Design review of the part built by this model. Coordinates are the model's own, in mm. Give positions to 0.01 mm unless a question says otherwise; leave off trailing zeros. Loops run counter-clockwise (first coordinate to the right, second up) from the corner with the lowest first, then second, coordinate; pieces in that order, holes last. Notation, with made-up numbers: M 61.5,-8.5 L 74.5,-8.5 A26 ccw 74.5,24.5 Z; hole C 27.5,35.25 d1. An arc over 180 degrees is marked long. Use one line per item in the form item = value. Start each with the question number.
from build123d import *

# Parameters (mm, degrees)
SKETCH1_W           = 25.4
SKETCH1_H           = 25.4
BOSS_EXTRUDE1_DEPTH = 3.175
CUT_EXTRUDE1_REACH  = 5.175
SKETCH2_R           = 2.5527


with BuildPart() as part:
    # Sketch1 → Boss-Extrude1 (new body)
    with BuildSketch(Plane.XY):
        with Locations((12.7, 12.7)):
            Rectangle(SKETCH1_W, SKETCH1_H)
    extrude(amount=BOSS_EXTRUDE1_DEPTH)

    # Sketch2 → Cut-Extrude1 (cut, up to next)
    with BuildSketch(Plane(origin=(0, 0, 0), x_dir=(-1, 0, 0), z_dir=(0, 0, -1)), mode=Mode.PRIVATE) as cut_extrude1_sk1:
        with Locations((-12.7, 6.35)):
            Circle(SKETCH2_R)
    cut_extrude1_tool1 = extrude(cut_extrude1_sk1.sketch, amount=-CUT_EXTRUDE1_REACH, mode=Mode.PRIVATE) & part.part
    add(cut_extrude1_tool1.solids().sort_by_distance((12.7, 6.35, 0))[0], mode=Mode.SUBTRACT)
    # Sketch2 → Cut-Extrude1 (cut, up to next)
    with BuildSketch(Plane(origin=(0, 0, 0), x_dir=(-1, 0, 0), z_dir=(0, 0, -1)), mode=Mode.PRIVATE) as cut_extrude1_sk2:
        with Locations((-12.7, 19.05)):
            Circle(SKETCH2_R)
    cut_extrude1_tool2 = extrude(cut_extrude1_sk2.sketch, amount=-CUT_EXTRUDE1_REACH, mode=Mode.PRIVATE) & part.part
    add(cut_extrude1_tool2.solids().sort_by_distance((12.7, 19.05, 0))[0], mode=Mode.SUBTRACT)


solid = part.part
Q1. Wall thickness on probe 1 along Y at (x, z) = (12.7, 2); probe 2 along Y at (x, z) = (12, 0.4); probe 3 along X at (y, z) = (6.5, 2.55): over which ranges is each line inside the solid? List them lowest first.
Q2. Take a section at C-C on z = 2.4. Give the boundary of the cut face in (x, y).
Q3. Take a section at B-B on y = 19.05. Give the boundary of the cut face in (x, z) (3 decimals).
Q4. Take a section at A-A on x = 12.7. Give the boundary of the cut face in (y, z) (3 decimals), plus the area to 3 significant figures.
Q5. Take a section at D-D on y = 5.75. Give the boundary of the cut face in (x, z) (3 decimals), plus the area to 3 significant figures.
Response values:
q1.probe_1 = 0 to 3.8, 8.9 to 16.5, 21.6 to 25.4
q1.probe_2 = 0 to 3.9, 8.8 to 16.6, 21.5 to 25.4
q1.probe_3 = 0 to 10.15, 15.25 to 25.4
q2.outline = M 0,0 L 25.4,0 L 25.4,25.4 L 0,25.4 Z; hole C 12.7,6.35 d5.11; hole C 12.7,19.05 d5.11
q3.outline = M 0,0 L 10.147,0 L 10.147,3.175 L 0,3.175 Z; M 15.253,0 L 25.4,0 L 25.4,3.175 L 15.253,3.175 Z
q4.outline = M 0,0 L 3.797,0 L 3.797,3.175 L 0,3.175 Z; M 8.903,0 L 16.497,0 L 16.497,3.175 L 8.903,3.175 Z; M 21.603,0 L 25.4,0 L 25.4,3.175 L 21.603,3.175 Z
q4.area = 48.2 mm^2
q5.outline = M 0,0 L 10.219,0 L 10.219,3.175 L 0,3.175 Z; M 15.181,0 L 25.4,0 L 25.4,3.175 L 15.181,3.175 Z
q5.area = 64.9 mm^2
